```python
from build123d import *

# Parameters (mm, degrees)
F4_R     = 0.254
F6_DEPTH = 0.4318


with BuildPart() as f1:
    # F0 (on Right) → F1 (revolve)
    with BuildSketch(Plane.YZ):
        with BuildLine():
            Line((-0.8096426782, 0), (0, 0))
            Line((0, 0), (1.5875, 0))
            Line((1.5875, 0), (1.5875, 3.4925))
            Line((1.5875, 3.4925), (0, 3.4925))
            ThreePointArc((0, 3.4925), (-0.6045832289, 1.7925594492), (-0.8096426782, 0))
        make_face()
    revolve(axis=Axis((0, 9.1738495976, 0), (0, -1, 0)))

    # F2 (on Right) → F3 (revolve)
    with BuildSketch(Plane.YZ):
        Polygon((2.38125, 1.59258), (1.5875, 1.59258), (1.5875, 0), (8.4455, 0), (8.4455, 1.4467282238), (7.65175, 1.905), (2.69367, 1.905), align=None)
    revolve(axis=Axis((0, 8.9318295941, 0), (0, 1, 0)))

    # F4
    f4_edges = [f1.edges().sort_by_distance(p)[0] for p in [
        (0, 1.5875, -1.59258),
        (0, 2.38125, -1.59258),
    ]]
    fillet(f4_edges, radius=F4_R)

    # F5 (on Top) → F6 (cut, symmetric)
    with BuildSketch(Plane.XY):
        with BuildLine():
            Line((3.4925, -1.3970176782), (3.4925, 0.3809823218))
            ThreePointArc((3.4925, 0.3809823218), (0, 1.1747323218), (-3.4925, 0.3809823218))
            Line((-3.4925, 0.3809823218), (-3.4925, -1.3970176782))
            Line((-3.4925, -1.3970176782), (3.4925, -1.3970176782))
        make_face()
    extrude(amount=F6_DEPTH, both=True, mode=Mode.SUBTRACT)


solid = f1.part
```
Input: part model. Units: mm. Frame: model coordinates. A direction names the side the tool comes from. Coordinates: 2 decimals unless noted, no trailing zeros. Loops run counter-clockwise (first coordinate to the right, second up) from the corner with the lowest first, then second, coordinate; pieces in that order, holes last. Notation, with made-up numbers: M -30,-7.75 L -13,-7.75 A20 ccw -13,0.25 Z; hole C -32.75,63.25 d2. An arc over 180 degrees is marked long. Use a Markdown table: item, result. Add a question column.
1) Draft query along X for faces 4 (the flat face through (0, 0, 0.432)), 5 (the flat face through (0, 8.446, 0)), 6 (the cylindrical face through (-1.86, 5.14, -0.41)). Return one class per face: +X half, -X half, draft (parallel to the pull), parting line (faces both ways), or undercut.
2) Set-up query: faces 1 (the flat face through (0, 0, -0.432)), 2 (the cylindrical face through (0.48, 2.06, 1.52)), 3 (the cylindrical face through (-3.463, 0.783, -0.455)). Return all of +Z, -Z, +X, -X, +Y, -Y with unobstructed straight access to the full face (end or side cutting, diameter ignored); none if empty.
3) Pin query (flat end, axial travel): P1, Ø1.5, axis at x = 1, z = 2.5, coming from the -Y side; P2, Ø1, axis at x = 1.5, y = 0, coming from the +Z side; P3, Ø1.5, axis at x = 1.5, y = 1, coming from the +Z side. Return the tip coordinate at first contact, or that it passes through.
4) Line query: L1, parallel to Z at x = 0, y = 2; L2, parallel to Z at x = 0.75, y = 0.5; L3, parallel to Z at x = -0.25, y = 0.5. Output: solid intervals per line, ascending. Write a range as from..to.
5) Section A-A, the plane x = 2.5. Return the cut outline in (y, z), plus the area to 3 significant figures.
6) Section B-B, the plane y = 3. Return the cut outline in (x, z) (3 decimals).
Answer below:
| question | item | result |
|---|---|---|
| 1 | face 4 | undercut |
| 1 | face 5 | draft |
| 1 | face 6 | parting line |
| 2 | face 1 | -Y |
| 2 | face 2 | none |
| 2 | face 3 | +Y, -Y |
| 3 | P1 | y = -0.57 |
| 3 | P2 | z = 3.35 |
| 3 | P3 | z = 3.41 |
| 4 | L1 | -1.59..1.59 |
| 4 | L2 | -3.41..-0.43, 0.43..3.41 |
| 4 | L3 | -3.48..-0.43, 0.43..3.48 |
| 5 | outline | M -0.39,-0.43 A7.53 ccw 0,-2.44 L 1.59,-2.44 L 1.59,2.44 L 0,2.44 A7.53 ccw -0.39,0.43 L 0.78,0.43 L 0.78,-0.43 Z |
| 5 | area | 8.05 mm2 |
| 6 | outline | C 0,0 d3.81 |
